Could you check a few things on this model? Use its own coordinates, in mm. Face numbers are marked on the shaded views. A direction names the side the tool comes from. Give positions to 0.01 mm unless a question says otherwise; leave off trailing zeros. Loops run counter-clockwise (first coordinate to the right, second up) from the corner with the lowest first, then second, coordinate; pieces in that order, holes last. Notation, with made-up numbers: M 0,-14.5 L 22,-14.5 A8 ccw 22,-8.5 Z; hole C 20.5,41.25 d1. An arc over 180 degrees is marked long. Answer in a Markdown table with one row per item. Add a question column.
```python
from build123d import *

# Parameters (mm, degrees)
F0_W      = 50
F0_H      = 12.5
F1_DEPTH  = 8
F2_DEPTH  = 75
F4_DEPTH  = 8
F7_DEPTH  = 3
F8_DEPTH  = 1
F11_DEPTH = 3
F14_DEPTH = 3
F15_DEPTH = 8
F16_DEPTH = 8
F17_DEPTH = 8


# Not quite as in the source:
# - a feature names something its author has since deleted; it is built from what else it names


with BuildPart() as f1:
    # F0 (on Top) → F1 (new body)
    with BuildSketch(Plane.XY):
        Polygon((57.9695070384, 39.3207329262), (60.5095952989, 40.7487522591), (42.0179491924, 72.7772228311), (-42.0179491924, 72.7772228311), (-84.0358983849, 0), (-42.0179491924, -72.7772228311), (42.0179491924, -72.7772228311), (84.0358983849, 0), (65.5269237886, 32.0584843966), (65.5097997054, 32.0881441788), (62.870004896, 30.6039762231), (65.3204122546, 26.2455930623), (60.0654171506, 23.2910848888), (57.615009792, 27.6494680496), (55.164720758, 32.0079177338), (52.7144317239, 36.366367418), (50.2642610162, 40.7248836223), (55.5194165334, 43.6791064608), align=None)
        with Locations((0, 54.5829171234)):
            Rectangle(F0_W, F0_H, mode=Mode.SUBTRACT)
    extrude(amount=F1_DEPTH)

    # F0 (on Top) → F2 (join)
    with BuildSketch(Plane.XY):
        Polygon((-84.0358983849, 0), (-87.5, 0), (-43.75, -75.7772228311), (43.75, -75.7772228311), (63.1745123486, -42.1329805311), (68.1246734519, -33.5590499945), (87.5, 0), (84.0358983849, 0), (42.0179491924, -72.7772228311), (-42.0179491924, -72.7772228311), align=None)
    extrude(amount=F2_DEPTH)

    # F0 (on Top) → F4 (join)
    with BuildSketch(Plane.XY):
        Polygon((43.75, 75.7772228311), (-43.75, 75.7772228311), (-65.625, 37.8886114156), (-68.125, 33.5584843966), (-87.5, 0), (-84.0358983849, 0), (-42.0179491924, 72.7772228311), (42.0179491924, 72.7772228311), (60.5095952989, 40.7487522591), (63.1248363216, 42.2190219338), align=None)
    extrude(amount=F4_DEPTH)

    # F6 (on face) → F7 (join)
    with BuildSketch(Plane(origin=(0, -50.1312366318, 89.3836679776), x_dir=(1, 0, 0), z_dir=(0, 0.4891706574, -0.872188092))):
        Polygon((43.75, 29.4041920927), (0, 29.4041920927), (-43.75, 29.4041920927), (-42.01795, -57.4775522498), (42.01795, -57.4775522498), align=None)
    extrude(amount=F7_DEPTH)

    # F3 (on Front) → F8 (join)
    with BuildSketch(Plane.XZ):
        Polygon((-42.01795, 114.5), (0, 114.5), (42.01795, 114.5), (84.0359, 75), (87.5, 75), (42.01795, 117.5), (0, 117.5), (-42.01795, 117.5), (-87.5, 75), (-84.0359, 75), align=None)
    extrude(amount=F8_DEPTH)

    # F10 (on face) → F11 (join)
    with BuildSketch(Plane(origin=(-67.6846727043, -39.0777640058, 72.4338274863), x_dir=(0.7723629594, -0.3015876344, 0.5590173143), z_dir=(-0.6351814378, -0.3667221741, 0.6797495039))):
        Polygon((33.2314262259, 55.789645187), (-25.6554603702, 35.6104118215), (30.9888924807, -31.0804218073), align=None)
    extrude(amount=-F11_DEPTH)

    # F13 (on face) → F14 (join)
    with BuildSketch(Plane(origin=(67.6756688636, -39.5950852503, 72.4241918832), x_dir=(0.7733047167, 0.3041472681, -0.556322078), z_dir=(-0.6340345536, 0.3709553614, -0.6785221475))):
        Polygon((-30.939509805, 30.5117392321), (-32.8751652468, -56.3649154418), (25.9400068576, -35.9776056011), align=None)
    extrude(amount=F14_DEPTH)

    # F0 (on Top) → F15 (join)
    with BuildSketch(Plane.XY):
        with Locations((0, 54.5829171234)):
            Rectangle(F0_W, F0_H)
    extrude(amount=F15_DEPTH)

    # F0 (on Top) → F16 (join)
    with BuildSketch(Plane.XY):
        Polygon((75.878553621, -32.3439069124), (73.3299584755, -36.6440801541), (78.4478092981, -39.6772904524), (80.9460908184, -35.4620099819), align=None)
        Polygon((73.3299584755, -36.6440801541), (68.1246734519, -33.5590499945), (63.1745123486, -42.1329805311), (68.2616414678, -45.1481695385), (73.3985163623, -48.1928433322), (78.4478092981, -39.6772904524), align=None)
        Polygon((73.3985163623, -48.1928433322), (68.2616414678, -45.1481695385), (65.7363801019, -49.4055813149), (70.880193178, -52.396181094), align=None)
    extrude(amount=F16_DEPTH)

    # F0 (on Top) → F17 (join)
    with BuildSketch(Plane.XY):
        Polygon((87.5, 0), (68.125, 33.5584843966), (65.5269237886, 32.0584843966), (84.0358983849, 0), align=None)
    extrude(amount=F17_DEPTH)


solid = f1.part
```
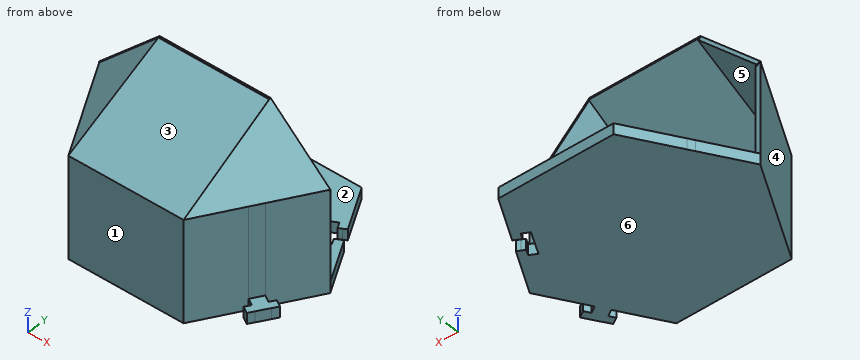
Item 1: Suppose I cut it at B-B (y = -29.5). List the corners of the cut face in (x, z) for me, then the cut area to 3 significant figures.
Item 2: I need wall thicknesses on L1, parallel to Z at x = 45, y = 49.5; L2, parallel to Y at x = 25.5, z = 42; L3, parallel to Z at x = 30.5, y = -2. Which ranges of each line are inside material? Lowest first, please.
Item 3: For the marked faces 1, 2 and 3, which set-ups out of +Z, -Z, +X, -X, +Y, -Y let a thin tool reach every point of the face, with its end or its side?
Item 4: For P1, Ø1, axis at x = 10, y = 31, coming from the +Z side; P2, Ø1.5, axis at x = 27.5, z = 26.5, coming from the +Y side; P3, Ø3, axis at y = -59, z = 77, coming from the +X side (3 decimals), each with a flat end and sliding along its axis, tell me the tip position at first contact or that it passes through.
Item 5: Suppose I cut it at D-D (z = 106.5). List the corners of the cut face in (x, y) for me.
Item 6: Suppose I cut it at C-C (z = 66.5). List the corners of the cut face in (x, y) for me, then the cut area to 3 significant figures.
Item 7: If we mould it in two halves opening along X, with no side actions, what happens to the marked faces 4, 5 and 6? For each: +X half, -X half, draft (parallel to the pull), parting line (faces both ways), or undercut.
Item 8: Suppose I cut it at A-A (x = 4.5). List the corners of the cut face in (y, z) for me, then the cut area to 3 significant figures.
Values found:
| question | item | result |
|---|---|---|
| 1 | outline | M -70.47,0 L 70.47,0 L 70.47,75 L 70.66,75.15 L 42.83,101.16 L 42.69,100.95 L -42.69,100.95 L -70.47,75 Z; hole M -67,8 L 67,8 L 67,74.15 L 42,97.52 L -41.65,97.52 L -67,73.82 Z |
| 1 | area | 2,110 mm² |
| 2 | L1 | 0 to 8 |
| 2 | L2 | -75.78 to -72.78 |
| 2 | L3 | 0 to 8, 112.94 to 116.38 |
| 3 | face 1 | +Z, -Z, +X, -X, -Y |
| 3 | face 2 | +Y |
| 3 | face 3 | +Z, -X, -Y |
| 4 | P1 | z = 8 |
| 4 | P2 | y = -72.78 |
| 4 | P3 | x = 53.255 |
| 5 | outline | M -53.79,-1 L -53.21,-1 L -42.47,-19.61 L 42.47,-19.61 L 42.65,-20.04 L 54.29,-0.14 L 50.21,0.98 L 41.76,-13.48 L -41.28,-13.48 L -49.7,1.1 L -53.79,0 Z |
| 6 | outline | M -87.5,0 L -43.75,-75.78 L 43.75,-75.78 L 87.5,0 L 84.04,0 L 42.02,-72.78 L -42.02,-72.78 L -84.04,0 Z |
| 6 | area | 772 mm² |
| 7 | face 4 | -X half |
| 7 | face 5 | undercut |
| 7 | face 6 | draft |
| 8 | outline | M -75.78,0 L 75.78,0 L 75.78,8 L -72.78,8 L -72.78,73.24 L 1.47,114.88 L 0,117.5 L -1,117.5 L -1,116.94 L -75.78,75 Z |
| 8 | area | 1,670 mm² |
